Could you check a few things on this model? Use its own coordinates, in mm. A direction names the side the tool comes from. Give positions to 0.01 mm unless a question says otherwise; leave off trailing zeros. Loops run counter-clockwise (first coordinate to the right, second up) from the corner with the lowest first, then second, coordinate; pieces in that order, holes last. Notation, with made-up numbers: (30, 85) - (36, 85) arc R24 ccw to (36, 116) - close; hole circle Ø10 at (53.25, 76.5). An arc over 180 degrees is marked (long way). Write each question's results on one line, items separated by ' | '. Start each with the question number.
1) I want a section at D-D, the plane y = -164.5. Write out the boundary of the cut face in (x, z).
2) I want a section at A-A, the plane z = 233.5. Write out the boundary of the cut face in (x, y).
3) I want a section at C-C, the plane y = -56.5. Write out the boundary of the cut face in (x, z).
4) I'm going to push flat-ended pins straight in: pin 1 (7.5 mm diameter, centred on x = 50.8, z = 50.8, fed in from +Y); pin 2 (1 mm diameter, centred on x = 123, z = 181, fed in from +Y); pin 3 (8 mm diameter, centred on x = 43.5, y = -25, fed in from -Z); pin 4 (19 mm diameter, centred on y = -115.5, z = 142.5, fed in from +X). Where does each tip first touch, or does it pass through?
5) On a 3-axis mill with a long thin cutter (end or side, diameter ignored), from which of +Z, -Z, +X, -X, +Y, -Y can I reach the whole of each face in a straight line? I mean faces 1 (the face through (14.486, -1.309, 15.276)), 2 (the face through (90, -152, 169.951)), 3 (the face through (139.7, 1, 151)). Say none if no direction works.
6) If we mould it in two halves opening along Z, with no side actions, what happens to faces 4 (the face through (5.73, -58.07, 150.98)), 5 (the face through (76, 1, 12.7)), 6 (the face through (76.56, 45.79, 5.15))? For each: +Z half, -Z half, draft (parallel to the pull), parting line (faces both ways), or undercut.
7) I want a section at B-B, the plane x = 65.5. Write out the boundary of the cut face in (y, z), and give its area (3 significant figures).
8) If I drill on probe 1 along Z at (x, y) = (90.5, -32); probe 2 along X at (y, z) = (-37, 60.5); probe 3 along Z at (x, y) = (50.8, -59.25), over which ranges is the centre line in solid material (lowest first)? Write a range as [from, to].
from build123d import *

# Parameters (mm, degrees)
F0_W      = 152.4
F0_H      = 50.8
F1_DEPTH  = 304.8
F2_R      = 50.8
F3_DEPTH  = 63.5
F4_T      = -12.7
F9_SIZE   = 10.16
F10_R     = 6.35
F5_DEPTH  = 114.301
F7_R      = 19.05
F6_W      = 25.2215266228
F6_H      = 63.5711848736
F11_DEPTH = 180.3614813834


# Not quite as in the source:
# - a feature names something its author has since deleted; it is built from what else it names


with BuildPart() as f1:
    # F0 (on Top) → F1 (new body)
    with BuildSketch(Plane.XY):
        with Locations((76.2, 25.4)):
            Rectangle(F0_W, F0_H)
    extrude(amount=F1_DEPTH)

    # F2
    f2_edges = [f1.edges().sort_by_distance(p)[0] for p in [
        (152.4, 25.4, 304.8),
        (152.4, 25.4, 0),
        (0, 25.4, 304.8),
        (0, 25.4, 0),
    ]]
    fillet(f2_edges, radius=F2_R)

    # F3 (add): a face of the model
    f3_faces = [f1.faces().sort_by_distance(p)[0] for p in [
        (76.2, 0, 152.4),
    ]]
    extrude(f3_faces, amount=F3_DEPTH)

    # F4
    f4_openings = [f1.faces().sort_by_distance(p)[0] for p in [
        (76.2, 50.8, 152.4),
    ]]
    offset(amount=F4_T, openings=f4_openings)

    # F9
    f9_edges = [f1.edges().sort_by_distance(p)[0] for p in [
        (0, 50.8, 152.4),
        (14.878976, 50.8, 14.878976),
        (137.521024, 50.8, 14.878976),
        (152.4, 50.8, 152.4),
        (137.521024, 50.8, 289.921024),
        (76.2, 50.8, 304.8),
        (76.2, 50.8, 0),
        (14.878976, 50.8, 289.921024),
    ]]
    chamfer(f9_edges, length=F9_SIZE)

    # F10 (on face) → F5 (cut, through all)
    with BuildSketch(Plane(origin=(0, 50.8, 0), x_dir=(-1, 0, 0), z_dir=(0, 1, 0))):
        with Locations((-50.8, 50.8)):
            Circle(F10_R)
    extrude(amount=-F5_DEPTH, mode=Mode.SUBTRACT)

    # F7
    f7_edges = [f1.edges().sort_by_distance(p)[0] for p in [
        (152.4, -63.5, 152.4),
        (0, -63.5, 152.4),
        (14.878976, -63.5, 289.921024),
        (14.878976, -63.5, 14.878976),
        (76.2, -63.5, 0),
        (76.2, -63.5, 304.8),
        (137.521024, -63.5, 14.878976),
        (137.521024, -63.5, 289.921024),
    ]]
    fillet(f7_edges, radius=F7_R)

    # F6 (on face) → F11 (join)
    with BuildSketch(Plane.XZ.offset(63.5)):
        with Locations((90.0648534298, 138.1654888391)):
            Rectangle(F6_W, F6_H)
    extrude(amount=F11_DEPTH)


solid = f1.part
Answers:
1) outline: (77.45, 106.38) - (102.68, 106.38) - (102.68, 169.95) - (77.45, 169.95) - close
2) outline: (0, -44.45) arc R19.05 ccw to (19.05, -63.5) - (133.35, -63.5) arc R19.05 ccw to (152.4, -44.45) - (152.4, 40.64) - (142.24, 50.8) - (139.7, 50.8) - (139.7, -50.8) - (12.7, -50.8) - (12.7, 50.8) - (10.16, 50.8) - (0, 40.64) - close
3) outline: (4.3, 50.8) arc R46.5 ccw to (50.8, 4.3) - (101.6, 4.3) arc R46.5 ccw to (148.1, 50.8) - (148.1, 254) arc R46.5 ccw to (101.6, 300.5) - (50.8, 300.5) arc R46.5 ccw to (4.3, 254) - close; hole circle Ø12.7 at (50.8, 50.8)
4) pin 1: passes through | pin 2: stops at y = -50.8 | pin 3: stops at z = 0.11 | pin 4: stops at x = 102.68
5) face 1: -Z, -X, +Y, -Y | face 2: +Z, +X, -X, -Y | face 3: +Y
6) face 4: draft | face 5: undercut | face 6: -Z half
7) outline: (-63.5, 19.05) arc R19.05 ccw to (-44.45, 0) - (40.64, 0) - (50.8, 10.16) - (50.8, 12.7) - (-50.8, 12.7) - (-50.8, 292.1) - (50.8, 292.1) - (50.8, 294.64) - (40.64, 304.8) - (-44.45, 304.8) arc R19.05 ccw to (-63.5, 285.75) - close | area: 6,190 mm2
8) probe 1: z = [0, 12.7], [292.1, 304.8] | probe 2: x = [0, 12.7], [139.7, 152.4] | probe 3: z = [7.06, 44.45], [57.15, 297.74]
